from build123d import *

# Parameters (mm, degrees)
F1_DEPTH      = 15
F2_DEPTH      = 7
F6_DEPTH      = 10
F6_DEPTH_BACK = 7
F5_R          = 2.25
F7_DEPTH      = 12
F9_DEPTH      = 20


with BuildPart() as f1:
    # F0 (on Top) → F1 (new body)
    with BuildSketch(Plane.XY):
        with BuildLine():
            ThreePointArc((0, -5), (3.5355339059, -3.5355339059), (5, 0))
            ThreePointArc((5, 0), (0, 5), (-5, 0))
            Line((-5, 0), (0, 0))
            Line((0, 0), (0, -5))
        make_face()
        with BuildLine():
            Line((0, 0), (-5, 0))
            ThreePointArc((-5, 0), (-3.5355339059, -3.5355339059), (0, -5))
            Line((0, -5), (0, 0))
        make_face()
    extrude(amount=F1_DEPTH)

    # F0 (on Top) → F2 (join)
    with BuildSketch(Plane.XY):
        with BuildLine():
            ThreePointArc((0, -5), (-3.5355339059, -3.5355339059), (-5, 0))
            Line((-5, 0), (-20, 0))
            Line((-20, 0), (-20, -7.5))
            Line((-20, -7.5), (0, -7.5))
            Line((0, -7.5), (0, -5))
        make_face()
    extrude(amount=F2_DEPTH)

    # F3 (on Front) → F4 (revolve)
    with BuildSketch(Plane.XZ):
        Polygon((0, 24.7979589711), (-5, 15), (0, 15), align=None)
    revolve(axis=Axis((0, 0, 19.8989794856), (0, 0, -1)))

    # F5 (on face) → F6 (join, two sides)
    with BuildSketch(Plane.XY.offset(7)) as f6_sk:
        with BuildLine():
            ThreePointArc((0, -5), (-0.9013878189, -4.9180788932), (-1.7732385626, -4.675))
            ThreePointArc((-1.7732385626, -4.675), (-1.0368220677, -5.4602631376), (0, -5.75))
            Line((0, -5.75), (0, -5))
        make_face()
        with BuildLine():
            ThreePointArc((2, -3.75), (-0.4761947473, -1.8075174228), (-1.7732385626, -4.675))
            ThreePointArc((-1.7732385626, -4.675), (-0.9013878189, -4.9180788932), (0, -5))
            Line((0, -5), (0, -5.75))
            ThreePointArc((0, -5.75), (1.4142135624, -5.1642135624), (2, -3.75))
        make_face()
        with BuildLine():
            Line((-20, -5.75), (-20, -1.75))
            ThreePointArc((-20, -1.75), (-22, -3.75), (-20, -5.75))
        make_face()
        with BuildLine():
            ThreePointArc((-20, -5.75), (-18.5857864376, -5.1642135624), (-18, -3.75))
            ThreePointArc((-18, -3.75), (-18.5857864376, -2.3357864376), (-20, -1.75))
            Line((-20, -1.75), (-20, -5.75))
        make_face()
    extrude(amount=F6_DEPTH)
    extrude(f6_sk.sketch, amount=-F6_DEPTH_BACK)

    # F5 (on face) → F7 (join)
    with BuildSketch(Plane.XY.offset(7)):
        with Locations((-10, -3.75)):
            Circle(F5_R)
    extrude(amount=F7_DEPTH)

    # F8 (on face) → F9 (join, through all)
    with BuildSketch(Plane(origin=(-20, 0, 0), x_dir=(0, -1, 0), z_dir=(-1, 0, 0))):
        Polygon((3.75, 13.9005221426), (0, 7), (1.75, 7), (5.75, 7), (7.5, 7), align=None)
    extrude(amount=-F9_DEPTH)

    # F11 (on face) → F12 (revolve)
    with BuildSketch(Plane.XZ.offset(3.75)):
        Polygon((-20, 19.9933259094), (-22, 17), (-20, 17), align=None)
    revolve(axis=Axis((-20, -3.75, 18.7693270892), (0, 0, 1)))

    # F11 (on face) → F13 (revolve)
    with BuildSketch(Plane.XZ.offset(3.75)):
        Polygon((-10, 21.6809513237), (-12.25, 19), (-10, 19), align=None)
    revolve(axis=Axis((-10, -3.75, 21.5624834672), (0, 0, 1)))

    # F11 (on face) → F14 (revolve)
    with BuildSketch(Plane.XZ.offset(3.75)):
        Polygon((0, 20), (-2, 17), (0, 17), align=None)
    revolve(axis=Axis((0, -3.75, 19.2562113553), (0, 0, 1)))


solid = f1.part
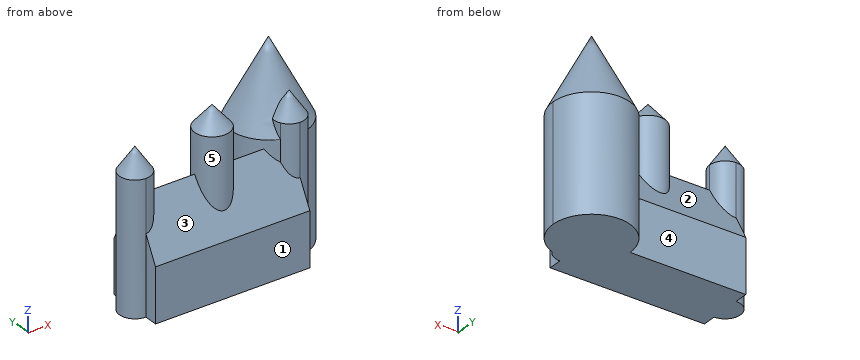
Here's how the part is built. I have some questions about the finished solid (model axes, mm). Face numbers are marked on the shaded views. A direction names the side the tool comes from. Round coordinates to 2 decimals unless told otherwise and drop trailing zeros. Loops run counter-clockwise (first coordinate to the right, second up) from the corner with the lowest first, then second, coordinate; pieces in that order, holes last. Notation, with made-up numbers: (69, -21) -> (102, -21) arc R27 ccw to (102, -1) -> close; hole circle Ø10 at (0.5, 48). An arc over 180 degrees is marked (long way). Write each question's results on one line, items separated by ' | '.
(1) If we section it at C-C, the plane z = 21: List the corners of the cut face in (x, y) for me, then the cut area to 3 significant figures.
Worked answers:
outline: circle Ø1.14 at (-10, -3.75); circle Ø3.88 at (0, 0) | area: 12.8 mm2
(2) If we section it at B-B, the plane x = -15.75: List the corners of the cut face in (y, z) for me, then the cut area to 3 significant figures.
Worked answers:
outline: (-7.5, 0) -> (0, 0) -> (0, 7) -> (-3.75, 13.9) -> (-7.5, 7) -> close | area: 78.4 mm2
(3) If we section it at D-D, the plane z = 18: List the corners of the cut face in (x, y) for me.
Worked answers:
outline: circle Ø2.66 at (-20, -3.75); circle Ø4.5 at (-10, -3.75); (-1.23, -3.24) arc R1.33 ccw (long way) to (1.23, -3.24) arc R3.47 ccw (long way) to start
(4) If we section it at A-A, the plane z = 3.25: List the corners of the cut face in (x, y) for me (3 decimals), then the cut area to 3 significant figures.
Worked answers:
outline: (-20, -7.5) -> (0, -7.5) -> (0, -5.75) arc R2 ccw to (1.773, -4.675) arc R5 ccw (long way) to (-5, 0) -> (-20, 0) -> (-20, -1.75) arc R2 ccw to (-20, -5.75) -> close | area: 216 mm2
(5) If I drill on L1, parallel to X at y = -2, z = 13.5; L2, parallel to Z at x = -18.75, y = -1.5; L3, parallel to Z at x = -19.5, y = -1, over which ranges is the centre line in solid material (lowest first)?
Worked answers:
L1: -20.97 to -19.03, -11.41 to -8.59, -4.58 to 4.58 | L2: 0 to 9.76 | L3: 0 to 8.84
(6) We'd pull the mould along X, two halves only. Please class the marked faces 1 and 2: released by +X, released by -X, zero draft, split by the parting line, or undercut.
Worked answers:
face 1: zero draft | face 2: undercut
(7) For the marked faces 3, 4 and 5, which set-ups out of +Z, -Z, +X, -X, +Y, -Y let a thin tool reach every point of the face, with its end or its side?
Worked answers:
face 3: +Z, -Y | face 4: +Z, -Z, -X, +Y | face 5: +Z
(8) For P1, Ø0.5, axis at y = -6.5, z = 6.5, coming from the -X side; P2, Ø0.9, axis at y = -6.5, z = 4.5, coming from the +X side; P3, Ø5, axis at x = -16, y = -4.5, coming from the +Z side, each with a flat end and sliding along its axis, tell me the tip position at first contact or that it passes through.
Worked answers:
P1: x = -20 | P2: x = 0 | P3: z = 17.64
